Source: CAD feature listing. Evaluate the final solid. Frame: model axes, mm. A direction names the side the tool comes from. Give positions to 0.01 mm unless a question says otherwise; leave off trailing zeros. Write each loop counter-clockwise with the first axis right and the second up, starting at its lowest first coordinate (ties: lowest second). Pieces come first, ordered by that corner, then holes. Notation, with made-up numbers: (28, 89.5) -> (45, 89.5) arc R21 ccw to (45, 111.5) -> close; hole circle Ø11 at (-25.5, -12). An arc over 180 degrees is marked (long way). Answer as a JSON object with one key per item and string values. Group by question number.
Item 1: Section query A-A on z = 2.75. Return the cut outline in (x, y), plus the area to 3 significant figures.
Item 2: Section query C-C on y = -6. Return the cut outline in (x, z), plus the area to 3 significant figures.
Item 3: Ray query, probe 1 along Z at (x, y) = (-24.5, -14); probe 2 along Y at (x, z) = (0, 0.6); probe 3 along X at (y, z) = (1, 1). Return the intervals inside material, ascending. Write a range as from..to.
Item 4: Pull-direction query (Y, two-part tool) for faces 3 (the face through (2.7, 2.8, 0.7)), 4 (the face through (3.625, -33.699, 0.74)), 5 (the face through (0.511, -32.453, 0.74)); classes: pulls with the +Y half, pulls with the -Y half, needs draft (parallel to the pull), parting line crosses it, or undercut.
Item 5: Section query D-D on x = -37. Give the number of separate pieces and of enclosed holes in the cut face, plus the area to 3 significant figures.
Item 6: Access query for faces 1 (the face through (-38, -17, 2)), 2 (the face through (-37, -17, 7)). Directions: +Z, -Z, +X, -X, +Y, -Y. A direction counts if a zero-diameter tool reaches every point of the face in a straight line with its end or side. Return the directions, or none.
Item 7: Section query B-B on x = -14. Return the cut outline in (y, z), plus the area to 3 significant figures.
Item 8: First-contact query: pin 1 Ø2.5 at (x, y) = (-37.5, -22) entering from -Z; pin 2 Ø8 at (x, y) = (-11.5, -26) entering from +Z. Flat tips, straight axial feed; report the tip coordinate or a pass-through.
from build123d import *

# Parameters (mm, degrees)
SKETCH_1_R      = 1.5
EXTRUDE_1_DEPTH = 1.5
SKETCH_2_W      = 5.5
SKETCH_2_H      = 12.5
EXTRUDE_2_DEPTH = 2
SKETCH_3_W      = 0.8
SKETCH_3_H      = 2
SKETCH_3_H_2    = 3
EXTRUDE_3_DEPTH = 4
SKETCH_4_W      = 0.5
SKETCH_4_H      = 0.5
EXTRUDE_4_DEPTH = 3


with BuildPart() as part:
    # 草图1 → 凸台-拉伸1 (new body)
    with BuildSketch(Plane.XY):
        with BuildLine():
            Line((-36.284526135, -8.481342061), (-35.853153699, -24.475525936))
            Line((-35.853153699, -24.475525936), (-35.662115389, -31.558736635))
            ThreePointArc((-35.662115389, -31.558736635), (-35.575705149, -31.939228692), (-35.350264491, -32.257689749))
            Line((-35.350264491, -32.257689749), (-30.305346266, -37.037625939))
            ThreePointArc((-30.305346266, -37.037625939), (-29.975196486, -37.245573186), (-29.590599895, -37.31134854))
            Line((-29.590599895, -37.31134854), (0.570005378, -36.497899484))
            ThreePointArc((0.570005378, -36.497899484), (0.950497435, -36.411489244), (1.268958491, -36.186048586))
            Line((1.268958491, -36.186048586), (6.048894681, -31.141130361))
            ThreePointArc((6.048894681, -31.141130361), (6.256841928, -30.810980581), (6.322617283, -30.42638399))
            Line((6.322617283, -30.42638399), (5.509168227, -0.265778718))
            ThreePointArc((5.509168227, -0.265778718), (5.422757987, 0.114713339), (5.197317328, 0.433174396))
            Line((5.197317328, 0.433174396), (0.152399104, 5.213110586))
            ThreePointArc((0.152399104, 5.213110586), (-0.177750677, 5.421057833), (-0.562347267, 5.486833187))
            Line((-0.562347267, 5.486833187), (-30.72295254, 4.673384131))
            ThreePointArc((-30.72295254, 4.673384131), (-31.103444597, 4.586973891), (-31.421905653, 4.361533233))
            Line((-31.421905653, 4.361533233), (-36.201841843, -0.683384991))
            ThreePointArc((-36.201841843, -0.683384991), (-36.40978909, -1.013534772), (-36.475564445, -1.398131363))
            Line((-36.475564445, -1.398131363), (-36.284526135, -8.481342061))
        make_face()
        with Locations((-30.988731257, -0.835784095)):
            Circle(SKETCH_1_R, mode=Mode.SUBTRACT)
        Circle(SKETCH_1_R, mode=Mode.SUBTRACT)
        with Locations((0.835784095, -30.988731257)):
            Circle(SKETCH_1_R, mode=Mode.SUBTRACT)
        with Locations((-30.152947162, -31.824515353)):
            Circle(SKETCH_1_R, mode=Mode.SUBTRACT)
    extrude(amount=EXTRUDE_1_DEPTH)

    # 草图2 → 凸台-拉伸2 (add)
    with BuildSketch(Plane(origin=(-36.486731964, -0.98406837, 0), x_dir=(0, 0, 1), z_dir=(-0.9996364921756676, -0.026960777264883006, 0))):
        with Locations((4.25, -15.5)):
            Rectangle(SKETCH_2_W, SKETCH_2_H)
    extrude(amount=-EXTRUDE_2_DEPTH)

    # 草图3 → 凸台-拉伸3 (add)
    with BuildSketch(Plane(origin=(-36.486731964, -0.98406837, 0), x_dir=(0, 0, 1), z_dir=(-0.9996364921756676, -0.026960777264883006, 0))):
        Polygon((2, -21.25), (2, -15.5), (1.5, -15.5), (1.5, -21.75), (5, -21.75), (5, -21.25), align=None)
        Polygon((1.5, -15.5), (2, -15.5), (2, -9.75), (5, -9.75), (5, -9.25), (1.5, -9.25), align=None)
        with Locations((6.6, -20.75)):
            Rectangle(SKETCH_3_W, SKETCH_3_H)
        with Locations((6.6, -17)):
            Rectangle(SKETCH_3_W, SKETCH_3_H_2)
        with Locations((6.6, -14)):
            Rectangle(SKETCH_3_W, SKETCH_3_H_2)
        with Locations((6.6, -10.25)):
            Rectangle(SKETCH_3_W, SKETCH_3_H)
    extrude(amount=EXTRUDE_3_DEPTH)

    # 草图4 → 凸台-拉伸4 (add)
    with BuildSketch(Plane(origin=(-36.486731964, -0.98406837, 0), x_dir=(0, 0, 1), z_dir=(-0.9996364921756676, -0.026960777264883006, 0))):
        with Locations((4.25, -19.822060647)):
            Rectangle(SKETCH_4_W, SKETCH_4_H)
        with Locations((4.25, -17.198296527)):
            Rectangle(SKETCH_4_W, SKETCH_4_H)
        with Locations((4.25, -13.801703473)):
            Rectangle(SKETCH_4_W, SKETCH_4_H)
        with Locations((4.25, -11.177939353)):
            Rectangle(SKETCH_4_W, SKETCH_4_H)
    extrude(amount=EXTRUDE_4_DEPTH)


solid = part.part
Worked answers:
{
 "1": {"outline": "(-40.24, -10.34) -> (-40.22, -10.84) -> (-36.22, -10.73) -> (-35.91, -22.23) -> (-39.91, -22.33) -> (-39.9, -22.83) -> (-33.9, -22.67) -> (-34.24, -10.18) -> close", "area": "29.0 mm^2"},
 "2": {"outline": "(-36.35, 0) -> (5.66, 0) -> (5.66, 1.5) -> (-36.35, 1.5) -> close", "area": "63.0 mm^2"},
 "3": {"probe 1": "0..1.5", "probe 2": "-36.51..-32.23, -29.74..-1.5, 1.5..5.33", "probe 3": "-34.61..-1.12, 1.12..4.6"},
 "4": {"face 3": "pulls with the +Y half", "face 4": "pulls with the -Y half", "face 5": "undercut"},
 "5": {"separate pieces": "8", "enclosed holes": "0", "area": "18.3 mm^2"},
 "6": {"face 1": "-X", "face 2": "+Z, +X, -X, +Y, -Y"},
 "7": {"outline": "(-36.89, 0) -> (5.12, 0) -> (5.12, 1.5) -> (-36.89, 1.5) -> close", "area": "63.0 mm^2"},
 "8": {"pin 1": "z = 1.5", "pin 2": "z = 1.5"}
}
